```python
from build123d import *

# Parameters (mm, degrees)
F0_W     = 20
F0_H     = 20
F1_DEPTH = 10
F2_R     = 5
F3_R     = 9.99999
F5_D     = 6
F7_D     = 12


# Not quite as in the source:
# - a fillet or chamfer is up to 0.001 mm smaller than in the source, because OpenCascade refuses the exact size


with BuildPart() as f1:
    # F0 (on Front) → F1 (new body)
    with BuildSketch(Plane.XZ):
        Polygon((-54.7173006759, -1.0133752964), (-14.7173006759, -1.0133752964), (-14.7173006759, 58.9866247036), (-54.7173006759, 58.9866247036), (-54.7173006759, 38.9866247036), (-54.7173006759, 18.9866247036), align=None)
        with Locations((-64.7173006759, 28.9866247036)):
            Rectangle(F0_W, F0_H)
    extrude(amount=F1_DEPTH)

    # F2
    f2_edges = [f1.edges().sort_by_distance(p)[0] for p in [
        (-54.717301, -5, 58.986625),
        (-54.717301, -5, -1.013375),
        (-14.717301, -5, 58.986625),
        (-14.717301, -5, -1.013375),
        (-54.717301, -5, 18.986625),
        (-54.717301, -5, 38.986625),
    ]]
    fillet(f2_edges, radius=F2_R)

    # F3 (radius 10 in the source; OpenCascade refuses exactly that, so slightly less here)
    f3_edges = [f1.edges().sort_by_distance(p)[0] for p in [
        (-74.717301, -5, 38.986625),
        (-74.717301, -5, 18.986625),
    ]]
    fillet(f3_edges, radius=F3_R)

    # F5 (through all)
    with Locations(Plane.XZ.offset(10)):
        with Locations((-44.7173006759, 48.9866247036), (-24.7173006759, 48.9866247036), (-24.7173006759, 8.9866247036), (-44.7173006759, 8.9866247036)):
            Hole(F5_D / 2)

    # F7 (through all)
    with Locations(Plane.XZ.offset(10)):
        with Locations((-64.7173006759, 28.9866247036)):
            Hole(F7_D / 2)


solid = f1.part
```
Source: CAD feature listing. Evaluate the final solid. Frame: model axes, mm. A direction names the side the tool comes from. Coordinates: 2 decimals unless noted, no trailing zeros. Loops run counter-clockwise (first coordinate to the right, second up) from the corner with the lowest first, then second, coordinate; pieces in that order, holes last. Notation, with made-up numbers: (72, -22.5) -> (100, -22.5) arc R27 ccw to (100, 4.5) -> close; hole circle Ø8 at (-30.5, -13). An arc over 180 degrees is marked (long way). One line per item, written item: value. Start each with the question number.
Q1. Set-up query: faces 4 (the face through (-54.717, -5, 49)), 5 (the face through (-41.72, -4.93, 9.12)), 6 (the face through (-62, -5, 18.987)). Return all of +Z, -Z, +X, -X, +Y, -Y with unobstructed straight access to the full face (end or side cutting, diameter ignored); none if empty.
Q2. Section query B-B, the plane x = -25.5. Return the cut outline in (y, z).
Q3. Section query A-A, the plane z = 31. Return the cut outline in (x, y).
Q4. Contact query for flat-ended pins moving along their axis: P1, Ø3, axis at y = -4.5, z = 7.5, coming from the -X side; P2, Ø5.5, axis at x = -62, y = -3.5, coming from the -Z side; P3, Ø2.5, axis at x = -63, y = -5.5, coming from the +Z side. Output: stop coordinate, or through.
Q5. Line query: line 1 along Z through (x, y) = (-26, -6.75); line 2 along Z through (x, y) = (-22.5, -9); line 3 along X through (y, z) = (-4.75, 4). Output: solid intervals per line, ascending.
Q6. Section query C-C, the plane z = 47. Return the cut outline in (x, y).
Q7. Section query D-D, the plane x = -61. Return the cut outline in (y, z).
Q8. Mould query, pull axis X, two halves, no side actions, for faces 1 (the face through (-71.866, -5.07, 35.98)), 2 (the face through (-38, -10, 29)), 3 (the face through (-42.34, -4.93, 47.16)). Classes: pulls with the +X half, pulls with the -X half, needs draft (parallel to the pull), parting line crosses it, or undercut.
Results:
1. face 4: +Z, -X, +Y, -Y
1. face 5: +Y, -Y
1. face 6: -Z, -X, +Y, -Y
2. outline: (-10, -1.01) -> (0, -1.01) -> (0, 6.09) -> (-10, 6.09) -> close; (-10, 11.88) -> (0, 11.88) -> (0, 46.09) -> (-10, 46.09) -> close; (-10, 51.88) -> (0, 51.88) -> (0, 58.99) -> (-10, 58.99) -> close
3. outline: (-74.51, -10) -> (-70.37, -10) -> (-70.37, 0) -> (-74.51, 0) -> close; (-59.07, -10) -> (-14.72, -10) -> (-14.72, 0) -> (-59.07, 0) -> close
4. P1: x = -54.72
4. P2: z = 18.96
4. P3: z = 38.99
5. line 1: -1.01 to 6.27, 11.7 to 46.27, 51.7 to 58.99
5. line 2: -1.01 to 6.97, 11.01 to 46.97, 51.01 to 58.99
5. line 3: -54.72 to -14.72
6. outline: (-54.72, -10) -> (-46.97, -10) -> (-46.97, 0) -> (-54.72, 0) -> close; (-42.47, -10) -> (-26.97, -10) -> (-26.97, 0) -> (-42.47, 0) -> close; (-22.47, -10) -> (-14.72, -10) -> (-14.72, 0) -> (-22.47, 0) -> close
7. outline: (-10, 18.99) -> (0, 18.99) -> (0, 24.28) -> (-10, 24.28) -> close; (-10, 33.7) -> (0, 33.7) -> (0, 38.99) -> (-10, 38.99) -> close
8. face 1: pulls with the -X half
8. face 2: needs draft
8. face 3: undercut
